Here's the drawing with two shaded views (mm, measured from the low corner). I have some questions. A direction names the side the tool comes from. Round coordinates to 2 decimals unless told otherwise and drop trailing zeros. Order: outer loops, then holes, each group sorted by start corner. A loop starts at its lowest first (then second) coordinate and runs counter-clockwise, first axis right, second up.
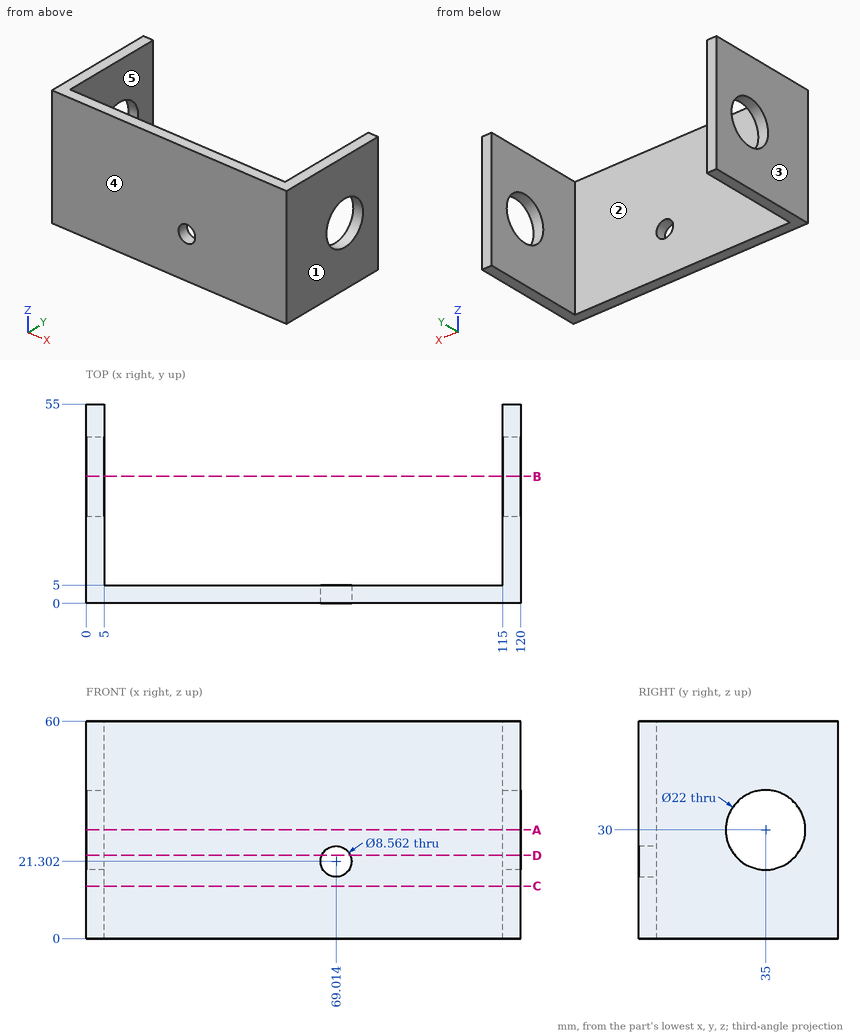
1. If we section it at D-D, the plane z = 23: Write out the boundary of the cut face in (x, y) (1 decimal).
Evaluation:
outline: (0, 0) - (65.1, 0) - (65.1, 5) - (5, 5) - (5, 26.5) - (0, 26.5) - close; (0, 43.5) - (5, 43.5) - (5, 55) - (0, 55) - close; (72.9, 0) - (120, 0) - (120, 26.5) - (115, 26.5) - (115, 5) - (72.9, 5) - close; (115, 43.5) - (120, 43.5) - (120, 55) - (115, 55) - close
2. On a 3-axis mill with a long thin cutter (end or side, diameter ignored), from which of +Z, -Z, +X, -X, +Y, -Y can I reach the whole of each face in a straight line? I mean the marked faces 1 and 2. Say none if no direction works.
Evaluation:
face 1: +Z, -Z, +X, +Y, -Y
face 2: +Z, -Z, +Y
3. I need wall thicknesses on probe 1 along X at (y, z) = (28, 47); probe 2 along Y at (x, z) = (118.4, 30); probe 3 along Y at (x, z) = (7.5, 45.5). Which ranges of each line are inside material? Lowest first, please.
Evaluation:
probe 1: x = 0 to 5, 115 to 120
probe 2: y = 0 to 24, 46 to 55
probe 3: y = 0 to 5
4. If we mould it in two halves opening along X, with no side actions, what happens to the marked faces 3, 4 and 5? For each: released by +X, released by -X, zero draft, split by the parting line, or undercut.
Evaluation:
face 3: released by -X
face 4: zero draft
face 5: undercut
5. If we section it at B-B, the plane y = 35: Write out the boundary of the cut face in (x, z).
Evaluation:
outline: (0, 0) - (5, 0) - (5, 19) - (0, 19) - close; (0, 41) - (5, 41) - (5, 60) - (0, 60) - close; (115, 0) - (120, 0) - (120, 19) - (115, 19) - close; (115, 41) - (120, 41) - (120, 60) - (115, 60) - close
6. I'm going to push a flat-ended pin straight in: P1, Ø4, axis at x = 97.5, z = 39.5, coming from the +Y side. Where does the tip first touch, or does it pass through?
Evaluation:
P1: stops at y = 5
7. If we section it at A-A, the plane z = 30: Write out the boundary of the cut face in (x, y), and give its area (3 significant figures).
Evaluation:
outline: (0, 0) - (120, 0) - (120, 24) - (115, 24) - (115, 5) - (5, 5) - (5, 24) - (0, 24) - close; (0, 46) - (5, 46) - (5, 55) - (0, 55) - close; (115, 46) - (120, 46) - (120, 55) - (115, 55) - close
area: 880 mm2
8. If we section it at C-C, the plane z = 14.5: Write out the boundary of the cut face in (x, y).
Evaluation:
outline: (0, 0) - (120, 0) - (120, 55) - (115, 55) - (115, 5) - (5, 5) - (5, 55) - (0, 55) - close
